Can you work these out from the model? Positions are in its coordinate system, mm. Coordinates: 2 decimals unless noted, no trailing zeros. Loops run counter-clockwise (first coordinate to the right, second up) from the corner with the lowest first, then second, coordinate; pieces in that order, holes last.
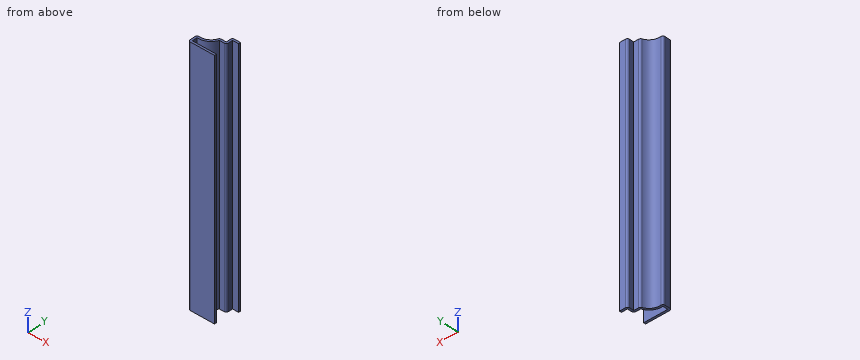
```python
from build123d import *

# Parameters (mm, degrees)
EXTRUDE_THIN1_DEPTH = 119.0625
FILLET1_R           = 1.016


with BuildPart() as part:
    # Sketch1 → Extrude-Thin1 (new body)
    with BuildSketch(Plane.XY):
        with BuildLine():
            Line((0, 0), (-12.7, 0))
            Line((-12.7, 0), (-12.7, 4.7625))
            ThreePointArc((-12.7, 4.7625), (-8.258259272, 5.18111669), (-5.55625, 8.73125))
            Line((-5.55625, 8.73125), (-2.38125, 8.73125))
            Line((-2.38125, 8.73125), (-2.38125, 11.90625))
            Line((-2.38125, 11.90625), (1.5875, 11.90625))
            Line((1.5875, 11.90625), (1.5875, 10.89025))
            Line((1.5875, 10.89025), (-1.36525, 10.89025))
            Line((-1.36525, 10.89025), (-1.36525, 7.71525))
            Line((-1.36525, 7.71525), (-4.8085569, 7.71525))
            ThreePointArc((-4.8085569, 7.71525), (-7.525174126, 4.432825355), (-11.684, 3.506279057))
            Line((-11.684, 3.506279057), (-11.684, 1.016))
            Line((-11.684, 1.016), (0, 1.016))
            Line((0, 1.016), (0, 0))
        make_face()
    extrude(amount=-EXTRUDE_THIN1_DEPTH)

    # Fillet1
    fillet1_edges = [part.edges().sort_by_distance(p)[0] for p in [
        (-1.36525, 7.71525, -59.53125),
        (-12.7, 0, -59.53125),
        (-12.7, 4.7625, -59.53125),
        (-5.55625, 8.73125, -59.53125),
        (-2.38125, 11.90625, -59.53125),
    ]]
    fillet(fillet1_edges, radius=FILLET1_R)


solid = part.part
```
(1) I want a section at C-C on y = 2. Write out the boundary of the cut face in (x, z).
Check values:
outline: (-12.7, -119.06) - (-11.68, -119.06) - (-11.68, 0) - (-12.7, 0) - close
(2) I want a section at B-B on z = -23. Write out the boundary of the cut face in (x, y).
Check values:
outline: (-12.7, 1.02) arc R1.02 ccw to (-11.68, 0) - (0, 0) - (0, 1.02) - (-11.68, 1.02) - (-11.68, 3.51) arc R6.57 ccw to (-4.81, 7.72) - (-2.38, 7.72) arc R1.02 ccw to (-1.37, 8.73) - (-1.37, 10.89) - (1.59, 10.89) - (1.59, 11.91) - (-1.37, 11.91) arc R1.02 ccw to (-2.38, 10.89) - (-2.38, 8.73) - (-4.81, 8.73) arc R1.02 ccw to (-5.76, 8.07) arc R5.56 cw to (-11.57, 4.52) arc R1.02 ccw to (-12.7, 3.51) - close
(3) I want a section at A-A on x = -9.75. Write out the boundary of the cut face in (y, z).
Check values:
outline: (0, -119.06) - (1.02, -119.06) - (1.02, 0) - (0, 0) - close; (3.58, -119.06) - (4.61, -119.06) - (4.61, 0) - (3.58, 0) - close
(4) I'm going to push flat-ended pins straight in: pin 1 (0.8 mm diameter, centred on y = 0.5, z = -50.5, fed in from +X); pin 2 (0.7 mm diameter, centred on y = 2, z = -42, fed in from +X); pin 3 (1.1 mm diameter, centred on y = 10, z = -66, fed in from -X). Where does each tip first touch, or does it pass through?
Check values:
pin 1: stops at x = 0
pin 2: stops at x = -11.68
pin 3: stops at x = -2.38
(5) If I drill on probe 1 along Y at (x, z) = (-2.5, -82); probe 2 along Y at (x, z) = (0.25, -56.5); probe 3 along Y at (x, z) = (-0.5, -85.5), over which ranges is the centre line in solid material (lowest first)?
Check values:
probe 1: y = 0 to 1.02, 7.72 to 8.73
probe 2: y = 10.89 to 11.91
probe 3: y = 0 to 1.02, 10.89 to 11.91
